```python
from build123d import *

# Parameters (mm, degrees)
CROQUIS1_R              = 1.5
CROQUIS1_R_2            = 1.25
CROQUIS1_RX             = 9
CROQUIS1_RY             = 6
SALIENTE_EXTRUIR1_DEPTH = 2.5


with BuildPart() as part:
    # Croquis1 → Saliente-Extruir1 (new body)
    with BuildSketch(Plane(origin=(0, 0, 0), x_dir=(1, 0, 0), z_dir=(0, 1, 0))):
        with BuildLine():
            Line((15, -30), (-18, -30))
            Line((-18, -30), (-32, -36.5))
            Line((-32, -36.5), (-68.831516336, -38.571772794))
            ThreePointArc((-68.831516336, -38.571772794), (-71.060891677, -37.756582308), (-72, -35.576507655))
            Line((-72, -35.576507655), (-72, 35.576507655))
            ThreePointArc((-72, 35.576507655), (-71.060891677, 37.756582308), (-68.831516336, 38.571772794))
            Line((-68.831516336, 38.571772794), (-32, 36.5))
            Line((-32, 36.5), (-18, 30))
            Line((-18, 30), (15, 30))
            ThreePointArc((15, 30), (17.121320344, 29.121320344), (18, 27))
            Line((18, 27), (18, -27))
            ThreePointArc((18, -27), (17.121320344, -29.121320344), (15, -30))
        make_face()
        with Locations((11.5, 24.5)):
            Circle(CROQUIS1_R, mode=Mode.SUBTRACT)
        with Locations((11.5, -24.5)):
            Circle(CROQUIS1_R, mode=Mode.SUBTRACT)
        with Locations((-9.25, 0)):
            Circle(CROQUIS1_R, mode=Mode.SUBTRACT)
        with Locations((-19.5, 18)):
            Circle(CROQUIS1_R_2, mode=Mode.SUBTRACT)
        with Locations((-19.5, -18)):
            Circle(CROQUIS1_R_2, mode=Mode.SUBTRACT)
        with Locations((-27.25, -14.25)):
            Circle(CROQUIS1_R, mode=Mode.SUBTRACT)
        with Locations((-27.25, 14.25)):
            Circle(CROQUIS1_R, mode=Mode.SUBTRACT)
        with Locations((-35.5, -33.944899023)):
            Circle(CROQUIS1_R, mode=Mode.SUBTRACT)
        with Locations((-46.5, -24.297446009)):
            Circle(CROQUIS1_R, mode=Mode.SUBTRACT)
        with Locations((-60.5, -33.598382655)):
            Circle(CROQUIS1_R, mode=Mode.SUBTRACT)
        with Locations((-35.5, 33.944899023)):
            Circle(CROQUIS1_R, mode=Mode.SUBTRACT)
        with Locations((-60.5, 33.598382655)):
            Circle(CROQUIS1_R, mode=Mode.SUBTRACT)
        with Locations((-46.5, 24.297446009)):
            Circle(CROQUIS1_R, mode=Mode.SUBTRACT)
        with Locations((-57.25, 14.25)):
            Circle(CROQUIS1_R, mode=Mode.SUBTRACT)
        with Locations((-69.5, 17.25)):
            Circle(CROQUIS1_R, mode=Mode.SUBTRACT)
        with Locations((-57.25, -14.25)):
            Circle(CROQUIS1_R, mode=Mode.SUBTRACT)
        with Locations((-69.5, -17.25)):
            Circle(CROQUIS1_R, mode=Mode.SUBTRACT)
        with Locations(Location((-42, 0), (0, 0, -90))):
            Ellipse(CROQUIS1_RX, CROQUIS1_RY, mode=Mode.SUBTRACT)
        with BuildLine():
            Line((7.5, 24.5), (7.5, 11.5))
            ThreePointArc((7.5, 11.5), (5.875, 9.875), (4.25, 11.5))
            Line((4.25, 11.5), (4.25, 24.5))
            ThreePointArc((4.25, 24.5), (5.875, 26.125), (7.5, 24.5))
        make_face(mode=Mode.SUBTRACT)
        with BuildLine():
            Line((7.5, -24.5), (7.5, -11.5))
            ThreePointArc((7.5, -11.5), (5.875, -9.875), (4.25, -11.5))
            Line((4.25, -11.5), (4.25, -24.5))
            ThreePointArc((4.25, -24.5), (5.875, -26.125), (7.5, -24.5))
        make_face(mode=Mode.SUBTRACT)
        with BuildLine():
            Line((-2.5, 24.5), (-2.5, 11.5))
            ThreePointArc((-2.5, 11.5), (-4.125, 9.875), (-5.75, 11.5))
            Line((-5.75, 11.5), (-5.75, 24.5))
            ThreePointArc((-5.75, 24.5), (-4.125, 26.125), (-2.5, 24.5))
        make_face(mode=Mode.SUBTRACT)
        with BuildLine():
            Line((-12.5, 24.5), (-12.5, 11.5))
            ThreePointArc((-12.5, 11.5), (-14.125, 9.875), (-15.75, 11.5))
            Line((-15.75, 11.5), (-15.75, 24.5))
            ThreePointArc((-15.75, 24.5), (-14.125, 26.125), (-12.5, 24.5))
        make_face(mode=Mode.SUBTRACT)
        with BuildLine():
            Line((-2.5, -24.5), (-2.5, -11.5))
            ThreePointArc((-2.5, -11.5), (-4.125, -9.875), (-5.75, -11.5))
            Line((-5.75, -11.5), (-5.75, -24.5))
            ThreePointArc((-5.75, -24.5), (-4.125, -26.125), (-2.5, -24.5))
        make_face(mode=Mode.SUBTRACT)
        with BuildLine():
            Line((-12.5, -24.5), (-12.5, -11.5))
            ThreePointArc((-12.5, -11.5), (-14.125, -9.875), (-15.75, -11.5))
            Line((-15.75, -11.5), (-15.75, -24.5))
            ThreePointArc((-15.75, -24.5), (-14.125, -26.125), (-12.5, -24.5))
        make_face(mode=Mode.SUBTRACT)
    extrude(amount=SALIENTE_EXTRUIR1_DEPTH)


solid = part.part
```
Work out the finished part from the listing and answer in its coordinate system (mm). A direction names the side the tool comes from. Coordinates: 2 decimals unless noted, no trailing zeros. Write each loop counter-clockwise with the first axis right and the second up, starting at its lowest first coordinate (ties: lowest second). Pieces come first, ordered by that corner, then holes.
Q1. Find the intervals of material crossed by line 1 (X direction, y = 1.1, z = 0); line 2 (X direction, y = 1.4, z = -14.25); line 3 (Z direction, x = -47, y = 1.1), in increasing order.
Q2. A cutting plane is placed at C-C, the plane z = 0. State how many separate pieces and enclosed holes the cut face has, then the cut area to 4 significant figures.
Q3. A cutting plane is placed at A-A, the plane x = 11.5. Give the vertices of the cut face in (y, z), then the cut area to 3 significant figures.
Q4. Which of the six approach directions +Z, -Z, +X, -X, +Y, -Y give full straight-line access (tool end or side, diameter ignored) to faces 4 (the face through (-4.089, 1.232, -9.875)), 5 (the face through (-50.16, 1.23, 37.52))?
Q5. A cutting plane is placed at B-B, the plane z = 14.25. Give the vertices of the cut face in (x, y).
Q6. Determine the mould class of faces 1 (the face through (-71.036, 1.232, 37.78)), 2 (the face through (18, 1, 0)), 3 (the face through (-18.345, 1.232, -17.521)) for opening direction Z: released by +Z, released by -Z, zero draft, split by the parting line, or undercut.
Q7. This flat-tipped pin is pushed along its axis until it touches: pin 1 Ø2 at (x, z) = (-19.5, 18) entering from -Y. Where does it stop, or does it pass through?
Findings below:
1. line 1: x = -72 to -48, -36 to -10.75, -7.75 to 18
1. line 2: x = -72 to -58.75, -55.75 to -28.75, -25.75 to -15.75, -12.5 to -5.75, -2.5 to 4.25, 7.5 to 18
1. line 3: z = -37.34 to -25.71, -22.88 to -4.97, 4.97 to 22.88, 25.71 to 37.34
2. separate pieces: 3
2. enclosed holes: 0
2. area: 187.5 mm2
3. outline: (0, -30) - (2.5, -30) - (2.5, -26) - (0, -26) - close; (0, -23) - (2.5, -23) - (2.5, 23) - (0, 23) - close; (0, 26) - (2.5, 26) - (2.5, 30) - (0, 30) - close
3. area: 135 mm2
4. face 4: +Y, -Y
4. face 5: +Z, +X, +Y, -Y
5. outline: (-72, 0) - (-58.75, 0) - (-58.75, 2.5) - (-72, 2.5) - close; (-55.75, 0) - (-28.75, 0) - (-28.75, 2.5) - (-55.75, 2.5) - close; (-25.75, 0) - (-15.75, 0) - (-15.75, 2.5) - (-25.75, 2.5) - close; (-12.5, 0) - (-5.75, 0) - (-5.75, 2.5) - (-12.5, 2.5) - close; (-2.5, 0) - (4.25, 0) - (4.25, 2.5) - (-2.5, 2.5) - close; (7.5, 0) - (18, 0) - (18, 2.5) - (7.5, 2.5) - close
6. face 1: released by +Z
6. face 2: zero draft
6. face 3: undercut
7. pin 1: passes through
